Answer from the drawing. Dimensions are ordinates in mm from the lowest x, y and z of the part. A direction names the side the tool comes from. Give positions to 0.01 mm unless a question says otherwise; leave off trailing zeros. Loops run counter-clockwise (first coordinate to the right, second up) from the corner with the lowest first, then second, coordinate; pieces in that order, holes last. Notation, with made-up numbers: (64.25, 26.5) - (74.25, 26.5) arc R10 cw to (74.25, 31.5) - close; hole circle Ø6 at (19, -2.5). An arc over 180 degrees is marked (long way). Write each question's results on one line, items separated by ' | '. Start each with the question number.
Q1. Determine the mould class of the marked faces 3, 4 and 5 for opening direction Z: +Z half, -Z half, draft (parallel to the pull), parting line (faces both ways), or undercut.
Q2. Given pin 1 (1.5 mm diameter, centred on x = 12.25, y = 20.5, fed in from +Z); pin 2 (2 mm diameter, centred on x = 12.25, y = 12.5, fed in from -Z), each flat-ended and moving along its own axis, determine where each tip first touches the part or whether it passes through.
Q3. The part is cut by section C-C, the plane z = 12. Write down the section's boundary in (x, y).
Q4. The part is cut by section B-B, the plane x = 23. Write down the section's boundary in (y, z), plus the area to 3 significant figures.
Q5. Find the intervals of material crossed by line 1 (Z direction, x = 33, y = 14.5); line 2 (X direction, y = 4.5, z = 36.6); line 3 (Y direction, x = 20.25, z = 36.1), in increasing order. Write a range as from..to.
Q6. For the marked faces 1 and 2, determine the directions among +Z, -Z, +X, -X, +Y, -Y from which every point of the face is accessible in a straight line to the end or side of a thin tool.
Q7. The part is cut by section A-A, the plane y = 12.5. State how many separate pieces and enclosed holes the cut face has, plus the area to 3 significant figures.
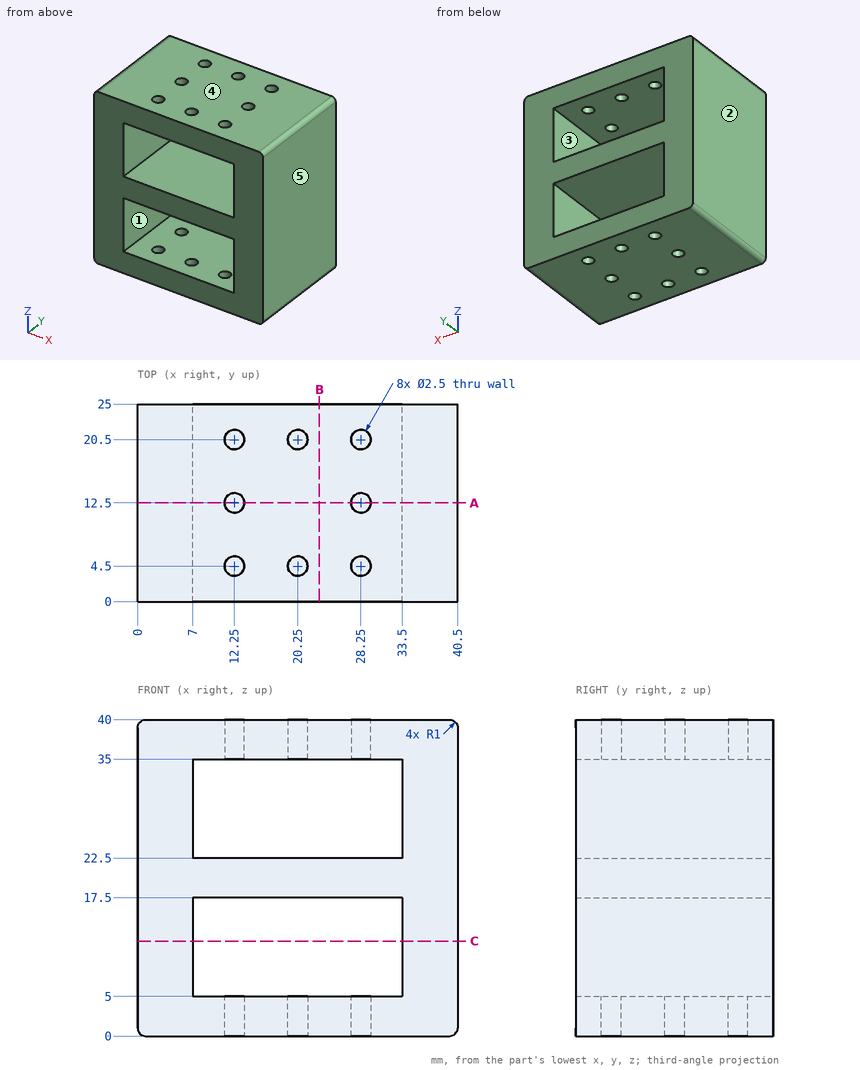
Check sheet entries:
1) face 3: undercut | face 4: +Z half | face 5: draft
2) pin 1: stops at z = 22.5 | pin 2: stops at z = 17.5
3) outline: (0, 0) - (7, 0) - (7, 25) - (0, 25) - close; (33.5, 0) - (40.5, 0) - (40.5, 25) - (33.5, 25) - close
4) outline: (0, 0) - (25, 0) - (25, 5) - (0, 5) - close; (0, 17.5) - (25, 17.5) - (25, 22.5) - (0, 22.5) - close; (0, 35) - (25, 35) - (25, 40) - (0, 40) - close | area: 375 mm^2
5) line 1: z = 0..5, 17.5..22.5, 35..40 | line 2: x = 0..11, 13.5..19, 21.5..27, 29.5..40.5 | line 3: y = 0..3.25, 5.75..19.25, 21.75..25
6) face 1: +Y, -Y | face 2: +Z, -Z, -X, +Y, -Y
7) separate pieces: 3 | enclosed holes: 0 | area: 907 mm^2
